Model file for the job. Use its own axes, mm. Round coordinates to 2 decimals unless told otherwise and drop trailing zeros. Loops run counter-clockwise (first coordinate to the right, second up) from the corner with the lowest first, then second, coordinate; pieces in that order, holes last. Notation, with made-up numbers: (-34, 58.25) - (0, 58.25) arc R11 ccw to (0, 69.25) - close; hole circle Ø11 at (-20.5, -1). An arc over 180 degrees is marked (long way). Answer as a JSON object with one key per item and string values.
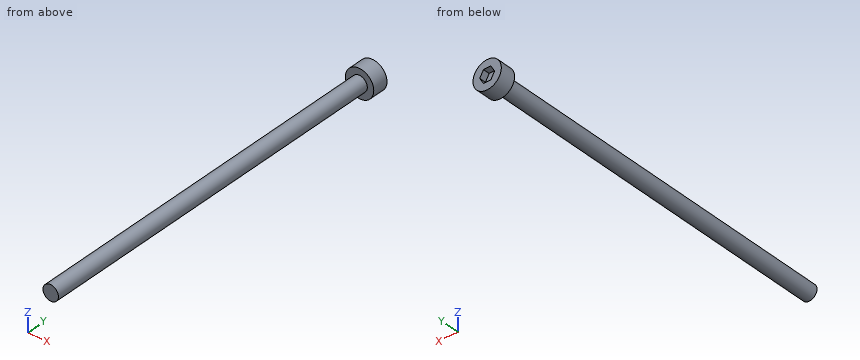
from build123d import *

# Parameters (mm, degrees)
SKETCH_1_R            = 2.75
EXTRUDE_248_DEPTH     = 3
CUT_EXTRUDE_378_DEPTH = 1.3
SKETCH_3_R            = 1.5
EXTRUDE_479_DEPTH     = 70


with BuildPart() as part:
    # 草图1 → Extrude 248 (new body)
    with BuildSketch(Plane(origin=(0, 0, 0), x_dir=(1, 0, 0), z_dir=(0, 1, 0))):
        Circle(SKETCH_1_R)
    extrude(amount=EXTRUDE_248_DEPTH)

    # 草图2 → Cut-Extrude 378 (cut)
    with BuildSketch(Plane(origin=(0, 3, 0), x_dir=(1, 0, 0), z_dir=(0, 1, 0))):
        Polygon((1.443375673, 0), (0.721687836, 1.25), (-0.721687836, 1.25), (-1.443375673, 0), (-0.721687836, -1.25), (0.721687836, -1.25), align=None)
    extrude(amount=-CUT_EXTRUDE_378_DEPTH, mode=Mode.SUBTRACT)

    # 草图3 → Extrude 479 (add)
    with BuildSketch(Plane.XZ):
        Circle(SKETCH_3_R)
    extrude(amount=EXTRUDE_479_DEPTH)


solid = part.part
1) Slice it at C-C on y = -44. List the corners of the cut face in (x, z).
Values follow:
{"outline": "circle Ø3 at (0, 0)"}
2) Slice it at A-A on x = 0. List the corners of the cut face in (y, z).
Values follow:
{"outline": "(-70, -1.5) - (0, -1.5) - (0, -2.75) - (3, -2.75) - (3, -1.25) - (1.7, -1.25) - (1.7, 1.25) - (3, 1.25) - (3, 2.75) - (0, 2.75) - (0, 1.5) - (-70, 1.5) - close"}
3) Drop flat-ended pins along their axis: P1, Ø1.5, axis at x = -1.5, y = -61, coming from the +Z side; P2, Ø1.5, axis at y = -21.5, z = 0, coming from the -X side; P3, Ø3, axis at y = -55, z = 0, coming from the +X side; P4, Ø1, axis at x = 0.5, y = 2, coming from the +Z side. Give the stop position or say it passes through.
Values follow:
{"P1": "z = 1.3", "P2": "x = -1.5", "P3": "x = 1.5", "P4": "z = 2.75"}
4) Probe probe 1 along Y at (x, z) = (0.15, -0.3); probe 2 along Y at (x, z) = (-0.1, 1.7); probe 3 along Z at (x, y) = (0, -17). List the from-to ranges inside material, lowest first.
Values follow:
{"probe 1": "-70 to 1.7", "probe 2": "0 to 3", "probe 3": "-1.5 to 1.5"}
5) Slice it at B-B on z = 0.6. List the corners of the cut face in (x, y).
Values follow:
{"outline": "(-2.68, 0) - (-1.37, 0) - (-1.37, -70) - (1.37, -70) - (1.37, 0) - (2.68, 0) - (2.68, 3) - (1.1, 3) - (1.1, 1.7) - (-1.1, 1.7) - (-1.1, 3) - (-2.68, 3) - close"}
